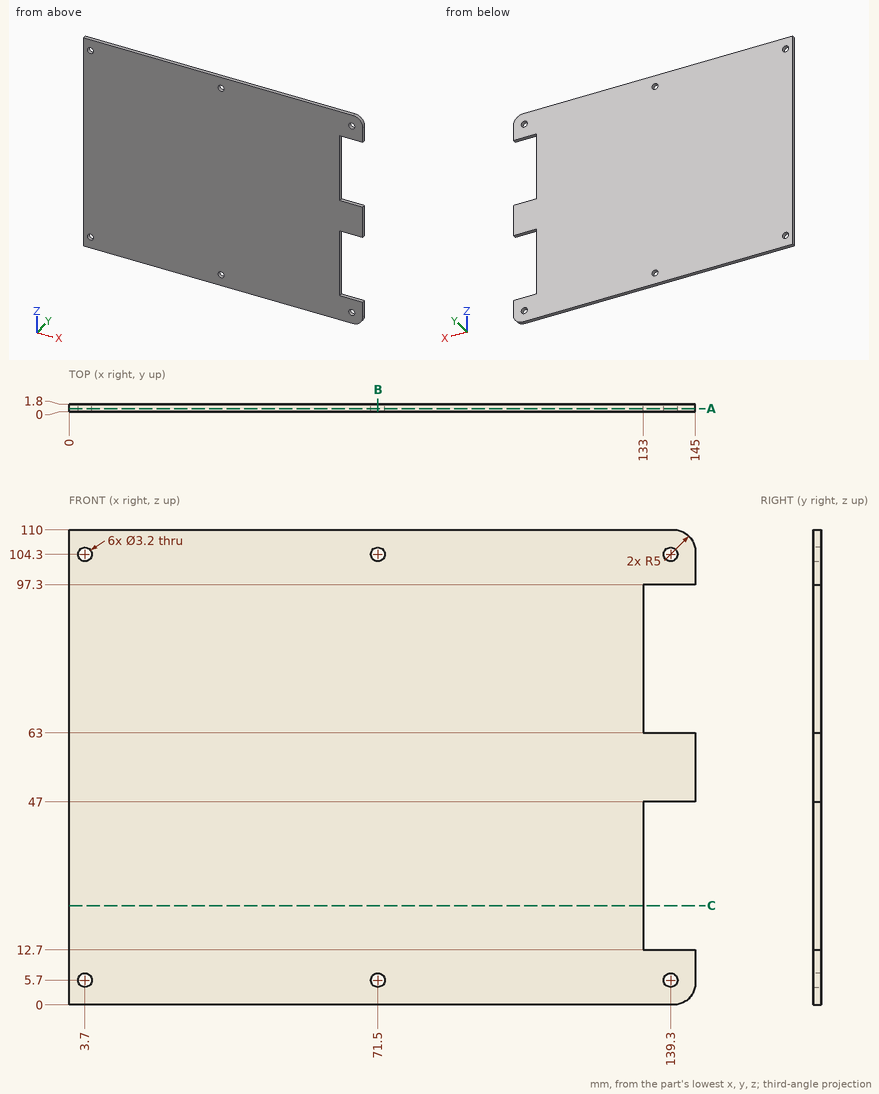
The figure shows three views and two pictorial views of one solid part (mm, origin at its lowest corner). Answer the questions. Coordinates: 2 decimals unless noted, no trailing zeros. Loops run counter-clockwise (first coordinate to the right, second up) from the corner with the lowest first, then second, coordinate; pieces in that order, holes last. Notation, with made-up numbers: (-38.5, 57) -> (-11.5, 57) arc R13 cw to (-11.5, 79) -> close; hole circle Ø8 at (27, -15). An arc over 180 degrees is marked (long way). Write item = value, one per line. Start each with the question number.
1) A cutting plane is placed at B-B (x = 71.5). Give the vertices of the cut face in (y, z).
2) A cutting plane is placed at C-C (z = 23). Give the vertices of the cut face in (x, y).
3) Straight lines are drawn through the part: line 1 (X direction, y = 1.4, z = 5.7); line 2 (Z direction, x = 139.3, y = 0.6); line 3 (Z direction, x = 71.5, y = 1.3). For each, find the intervals that lie inside material, in ascending order. Write a range as from..to.
4) Given pin 1 Ø2.5 at (x, z) = (139.3, 104.3) entering from +Y; pin 2 Ø1 at (y, z) = (1, 16.5) entering from -X; pin 3 Ø0.9 at (y, z) = (1.5, 27) entering from +X, each flat-ended and moving along its own axis, determine where each tip first touches the part or whether it passes through.
5) A cutting plane is placed at A-A (y = 0.75). Give the vertices of the cut face in (x, z), then the cut area to 3 significant figures.
Responses:
q1.outline = (0, 0) -> (1.8, 0) -> (1.8, 4.1) -> (0, 4.1) -> close; (0, 7.3) -> (1.8, 7.3) -> (1.8, 102.7) -> (0, 102.7) -> close; (0, 105.9) -> (1.8, 105.9) -> (1.8, 110) -> (0, 110) -> close
q2.outline = (0, 0) -> (133, 0) -> (133, 1.8) -> (0, 1.8) -> close
q3.line_1 = 0..2.1, 5.3..69.9, 73.1..137.7, 140.9..145
q3.line_2 = 0..4.1, 7.3..12.7, 47..63, 97.3..102.7, 105.9..110
q3.line_3 = 0..4.1, 7.3..102.7, 105.9..110
q4.pin_1 = through
q4.pin_2 = 0
q4.pin_3 = 133
q5.outline = (0, 0) -> (140, 0) arc R5 ccw to (145, 5) -> (145, 12.7) -> (133, 12.7) -> (133, 47) -> (145, 47) -> (145, 63) -> (133, 63) -> (133, 97.3) -> (145, 97.3) -> (145, 105) arc R5 ccw to (140, 110) -> (0, 110) -> close; hole circle Ø3.2 at (3.7, 5.7); hole circle Ø3.2 at (3.7, 104.3); hole circle Ø3.2 at (71.5, 5.7); hole circle Ø3.2 at (71.5, 104.3); hole circle Ø3.2 at (139.3, 5.7); hole circle Ø3.2 at (139.3, 104.3)
q5.area = 15,100 mm²
